Here's how the part is built. I have some questions about the finished solid (model axes, mm). Face numbers are marked on the shaded views. Coordinates: 2 decimals unless noted, no trailing zeros. Order: outer loops, then holes, each group sorted by start corner. A loop starts at its lowest first (then second) coordinate and runs counter-clockwise, first axis right, second up.
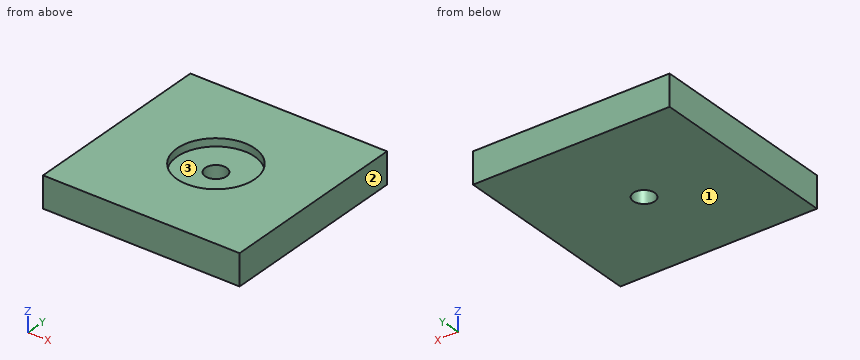
```python
from build123d import *

# Parameters (mm, degrees)
F0_W     = 50.484959
F0_H     = 50
F1_DEPTH = 8
F2_R     = 10
F3_DEPTH = 2
F4_R     = 2.75
F5_DEPTH = 6.001


with BuildPart() as f1:
    # F0 (on Top) → F1 (new body)
    with BuildSketch(Plane.XY):
        with Locations((-0.242479, 0)):
            Rectangle(F0_W, F0_H)
    extrude(amount=-F1_DEPTH)

    # F2 (on Top) → F3 (cut)
    with BuildSketch(Plane.XY):
        Circle(F2_R)
    extrude(amount=-F3_DEPTH, mode=Mode.SUBTRACT)

    # F4 (on face) → F5 (cut, through all)
    with BuildSketch(Plane.XY.offset(-2)):
        Circle(F4_R)
    extrude(amount=-F5_DEPTH, mode=Mode.SUBTRACT)


solid = f1.part
```
Q1. If we section it at B-B on x = 0: Write out the boundary of the cut face in (y, z).
Q2. If we section it at C-C on x = 6: Write out the boundary of the cut face in (y, z).
Q3. We'd pull the mould along X, two halves only. Please class the marked faces 1, 2 and 3: pulls with the +X half, pulls with the -X half, needs draft (parallel to the pull), parting line crosses it, or undercut.
Q4. I need wall thicknesses on L1, parallel to Y at x = 0, z = -0.8; L2, parallel to Y at x = 0, z = -4.2; L3, parallel to Z at x = 1, y = -4. Which ranges of each line are inside material? Lowest first, please.
Q5. If we section it at D-D on y = 5.5: Write out the boundary of the cut face in (x, z), then the cut area to 3 significant figures.
Q6. If we section it at A-A on y = 0: Write out the boundary of the cut face in (x, z), then the cut area to 3 significant figures.
Reply:
1. outline: (-25, -8) - (-2.75, -8) - (-2.75, -2) - (-10, -2) - (-10, 0) - (-25, 0) - close; (2.75, -8) - (25, -8) - (25, 0) - (10, 0) - (10, -2) - (2.75, -2) - close
2. outline: (-25, -8) - (25, -8) - (25, 0) - (8, 0) - (8, -2) - (-8, -2) - (-8, 0) - (-25, 0) - close
3. face 1: needs draft
3. face 2: pulls with the +X half
3. face 3: undercut
4. L1: y = -25 to -10, 10 to 25
4. L2: y = -25 to -2.75, 2.75 to 25
4. L3: z = -8 to -2
5. outline: (-25.48, -8) - (25, -8) - (25, 0) - (8.35, 0) - (8.35, -2) - (-8.35, -2) - (-8.35, 0) - (-25.48, 0) - close
5. area: 370 mm2
6. outline: (-25.48, -8) - (-2.75, -8) - (-2.75, -2) - (-10, -2) - (-10, 0) - (-25.48, 0) - close; (2.75, -8) - (25, -8) - (25, 0) - (10, 0) - (10, -2) - (2.75, -2) - close
6. area: 331 mm2
